Geometry: final body of the model. Coordinates: model frame, mm. Face numbers are marked on the shaded views. A direction names the side the tool comes from. Give positions to 0.01 mm unless a question says otherwise; leave off trailing zeros. Write each loop counter-clockwise with the first axis right and the second up, starting at its lowest first coordinate (ties: lowest second). Pieces come first, ordered by that corner, then holes. Notation, with made-up numbers: (8, 22) - (18, 22) arc R22 ccw to (18, 43) - close; hole circle Ø6 at (-23, -34.5). An arc over 180 degrees is marked (long way). Return JSON: item names as keys, results as strings.
from build123d import *

# Parameters (mm, degrees)
F1_DEPTH = 120
F3_DEPTH = 8
F5_DEPTH = 100
F6_W     = 908.2950688624
F6_H     = 128
F7_DEPTH = 12


with BuildPart() as f1:
    # F0 (on Top) → F1 (new body)
    with BuildSketch(Plane.XY):
        Polygon((802.5, -8.4689717992), (24.5, -268.4689717992), (24.5, -880), (802.5, -620), align=None)
    extrude(amount=F1_DEPTH)

    # F2 (on face) → F3 (cut)
    with BuildSketch(Plane(origin=(0, 0, 0), x_dir=(1, 0, 0), z_dir=(0, 0, -1))):
        Polygon((36.5, 277.1110551236), (790.5, 25.1316206763), (790.5, 611.3579166756), (36.5, 863.3373511229), align=None)
    extrude(amount=-F3_DEPTH, mode=Mode.SUBTRACT)

    # F4 (on face) → F5 (cut, through all)
    with BuildSketch(Plane.XY.offset(120)):
        Polygon((790.5, -611.3579166756), (790.5, -25.1316206763), (36.5, -277.1110551236), (36.5, -863.3373511229), align=None)
    extrude(amount=-F5_DEPTH, mode=Mode.SUBTRACT)

    # F6 (on face) → F7 (join, through all)
    with BuildSketch(Plane(origin=(267.0038223527, -798.9575915017, 0), x_dir=(0.9484392014, 0.3169591161, 0), z_dir=(0.3169591161, -0.9484392014, 0))):
        with Locations((177.4602726623, 60)):
            Rectangle(F6_W, F6_H)
    extrude(amount=-F7_DEPTH)


solid = f1.part
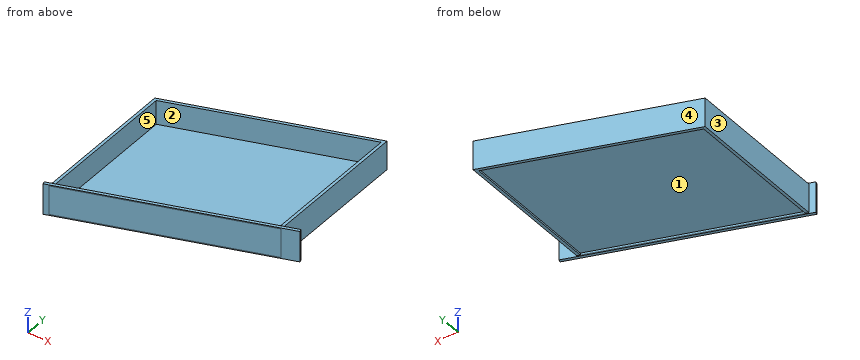
Q1. Material intervals for probe 1 along X at (y, z) = (-506.5, 52); probe 2 along Z at (x, y) = (469, -234.5); probe 3 along Y at (x, z) = (282, 67), sorted ascending. Write a range as [from, to].
Answer key:
{"probe 1": "x = [24.5, 36.5], [790.5, 802.5]", "probe 2": "z = [8, 20]", "probe 3": "y = [-793.95, -781.29], [-195.07, -182.41]"}
Q2. Set-up query: the marked faces 1 and 2. Return all of +Z, -Z, +X, -X, +Y, -Y with unobstructed straight access to the full face (end or side cutting, diameter ignored); none if empty.
Answer key:
{"face 1": "-Z", "face 2": "+Z"}
Q3. Pin query (flat end, axial travel): P1, Ø5, axis at x = 361, z = 26.5, coming from the -Y side; P2, Ø4, axis at y = -311, z = 5.5, coming from the -X side; P3, Ø2, axis at x = 423, z = 30.5, coming from the -Y side. Return the tip coordinate at first contact, or that it passes through.
Answer key:
{"P1": "stops at y = -768.38", "P2": "stops at x = 24.5", "P3": "stops at y = -747.16"}
Q4. Section query B-B, the plane y = -497. Return the cut outline in (x, z).
Answer key:
{"outline": "(24.5, 0) - (36.5, 0) - (36.5, 8) - (790.5, 8) - (790.5, 0) - (802.5, 0) - (802.5, 120) - (790.5, 120) - (790.5, 20) - (36.5, 20) - (36.5, 120) - (24.5, 120) - close"}
Q5. Section query D-D, the plane y = -727.5. Return the cut outline in (x, z).
Answer key:
{"outline": "(24.5, 0) - (36.5, 0) - (36.5, 8) - (442.97, 8) - (442.97, -4) - (480.83, -4) - (480.83, 124) - (442.97, 124) - (442.97, 20) - (36.5, 20) - (36.5, 120) - (24.5, 120) - close"}
Q6. Mould query, pull axis Y, two halves, no side actions, for the marked faces 3, 4 and 5. Classes: pulls with the +Y half, pulls with the -Y half, needs draft (parallel to the pull), parting line crosses it, or undercut.
Answer key:
{"face 3": "needs draft", "face 4": "pulls with the +Y half", "face 5": "undercut"}
Q7. Section query A-A, the plane z = 61. Return the cut outline in (x, y), plus the area to 3 significant figures.
Answer key:
{"outline": "(0.78, -875.27) - (4.58, -886.66) - (866.05, -598.76) - (862.24, -587.38) - (802.5, -607.35) - (802.5, -8.47) - (24.5, -268.47) - (24.5, -867.35) - close; hole (36.5, -863.34) - (790.5, -611.36) - (790.5, -25.13) - (36.5, -277.11) - close", "area": "34,800 mm^2"}
Q8. Section query C-C, the plane x = 88.5. Return the cut outline in (y, z), plus the area to 3 significant figures.
Answer key:
{"outline": "(-858.61, -4) - (-845.96, -4) - (-845.96, 8) - (-259.73, 8) - (-259.73, 0) - (-247.08, 0) - (-247.08, 120) - (-259.73, 120) - (-259.73, 20) - (-845.96, 20) - (-845.96, 124) - (-858.61, 124) - close", "area": "10,200 mm^2"}
